Could you check a few things on this model? Use its own coordinates, in mm. Coordinates: 2 decimals unless noted, no trailing zeros. Loops run counter-clockwise (first coordinate to the right, second up) from the corner with the lowest first, then second, coordinate; pieces in that order, holes last. Notation, with made-up numbers: (-33, 13.5) - (23, 13.5) arc R31 ccw to (23, 42.5) - close; hole circle Ø9 at (37.5, 55.25). An arc over 180 degrees is marked (long way). Use CSV: the item, a comma, the result in double quotes.
from build123d import *

# Parameters (mm, degrees)
F0_W           = 56.4960166812
F0_H           = 37.580087781
F1_DEPTH       = 25.4
F2_R           = 5.08
F4_D           = 6.35
F4_CSINK_D     = 12.7
F4_CSINK_ANGLE = 90


with BuildPart() as f1:
    # F0 (on Front) → F1 (new body)
    with BuildSketch(Plane.XZ):
        with Locations((28.2480083406, 18.7900438905)):
            Rectangle(F0_W, F0_H)
    extrude(amount=F1_DEPTH)

    # F2
    f2_edges = [f1.edges().sort_by_distance(p)[0] for p in [
        (56.496017, -12.7, 37.580088),
    ]]
    fillet(f2_edges, radius=F2_R)

    # F4 (through all)
    with Locations(Plane(origin=(0, 0, 0), x_dir=(1, 0, 0), z_dir=(0, 1, 0))):
        with Locations((8.5900304839, -31.4149707556), (6.8720257841, -10.3080365807), (36.81441769, -10.3080365807), (49.0858890116, -31.4149707556)):
            CounterSinkHole(F4_D / 2, F4_CSINK_D / 2, counter_sink_angle=F4_CSINK_ANGLE)


solid = f1.part
(1) Please list where these lines run through material, in increasing order: line 1 (X direction, y = -16.75, z = 31.5); line 2 (X direction, y = -9, z = 29.5); line 3 (Z direction, x = 4.5, y = -8).
Computed:
line 1,"x = 0 to 5.42, 11.76 to 45.91, 52.26 to 56.5"
line 2,"x = 0 to 6.06, 11.12 to 46.55, 51.62 to 56.5"
line 3,"z = 0 to 8.2, 12.42 to 37.58"
(2) Will this pin go through, and if not, where does the flat tip stop? pin 1 (5 mm diameter, centred on x = 36, z = 13, fed in from +Y).
Computed:
pin 1,"stops at y = -1.04"
(3) Suppose I cut it at B-B (z = 9). State how many separate pieces and enclosed holes the cut face has, plus the area to 3 significant figures.
Computed:
separate pieces,"3"
enclosed holes,"0"
area,"1,120 mm²"
(4) Suppose I cut it at A-A (y = -12.75). Write out the boundary of the cut face in (x, z) (3 decimals).
Computed:
outline,"(0, 0) - (56.496, 0) - (56.496, 32.5) arc R5.08 ccw to (51.416, 37.58) - (0, 37.58) - close; hole circle Ø6.35 at (6.872, 10.308); hole circle Ø6.35 at (8.59, 31.415); hole circle Ø6.35 at (36.814, 10.308); hole circle Ø6.35 at (49.086, 31.415)"
(5) Thinking about a two-plate mould opening in Z: for faces 1 (the face through (25, -13, 37.58)), 2 (the face through (5.4, -3, 30.4)), 3 (the face through (56.496, -13, 16)), which applies, +Z half, -Z half, draft (parallel to the pull), parting line (faces both ways), or undercut?
Computed:
face 1,"+Z half"
face 2,"undercut"
face 3,"draft"
